Could you check a few things on this model? Use its own coordinates, in mm. A direction names the side the tool comes from. Coordinates: 2 decimals unless noted, no trailing zeros. Loops run counter-clockwise (first coordinate to the right, second up) from the corner with the lowest first, then second, coordinate; pieces in that order, holes last. Notation, with made-up numbers: (54.5, -17.5) - (102.5, -17.5) arc R26 ccw to (102.5, 10.5) - close; hole circle Ø3 at (-20.75, 41). An arc over 180 degrees is marked (long way). Use CSV: the item, a comma, the result in double quotes.
from build123d import *

# Parameters (mm, degrees)
SKETCH1_W           = 80
SKETCH1_H           = 40
BOSS_EXTRUDE1_DEPTH = 100
CUT_EXTRUDE1_DEPTH  = 100
SKETCH4_W           = 20
SKETCH4_H           = 10
CUT_EXTRUDE2_DEPTH  = 100
SKETCH5_W           = 10
SKETCH5_H           = 40
CUT_EXTRUDE3_DEPTH  = 100
SKETCH7_R           = 5
BOSS_EXTRUDE2_DEPTH = 20


with BuildPart() as part:
    # Sketch1 → Boss-Extrude1 (new body)
    with BuildSketch(Plane(origin=(0, 0, 0), x_dir=(1, 0, 0), z_dir=(0, 1, 0))):
        Rectangle(SKETCH1_W, SKETCH1_H)
    extrude(amount=BOSS_EXTRUDE1_DEPTH)

    # Sketch2 → Cut-Extrude1 (cut)
    with BuildSketch(Plane.XY.offset(20)):
        with BuildLine():
            ThreePointArc((20, 30), (34.142135624, 24.142135624), (40, 10))
            Line((40, 10), (40, 100))
            Line((40, 100), (20, 100))
            Line((20, 100), (20, 90))
            ThreePointArc((20, 90), (-10, 60), (20, 30))
        make_face()
        with BuildLine():
            Line((-40, 100), (-40, 70))
            ThreePointArc((-40, 70), (-31.213203436, 91.213203436), (-10, 100))
            Line((-10, 100), (-40, 100))
        make_face()
    extrude(amount=-CUT_EXTRUDE1_DEPTH, mode=Mode.SUBTRACT)

    # Sketch4 → Cut-Extrude2 (cut)
    with BuildSketch(Plane(origin=(40, 0, 0), x_dir=(0, 0, -1), z_dir=(1, 0, 0))):
        with Locations((0, 5)):
            Rectangle(SKETCH4_W, SKETCH4_H)
    extrude(amount=-CUT_EXTRUDE2_DEPTH, mode=Mode.SUBTRACT)

    # Sketch5 → Cut-Extrude3 (cut)
    with BuildSketch(Plane(origin=(20, 0, 0), x_dir=(0, 0, -1), z_dir=(1, 0, 0))):
        with Locations((-15, 80)):
            Rectangle(SKETCH5_W, SKETCH5_H)
    extrude(amount=-CUT_EXTRUDE3_DEPTH, mode=Mode.SUBTRACT)

    # Sketch7 → Boss-Extrude2 (add)
    with BuildSketch(Plane(origin=(0, 0, 0), x_dir=(1, 0, 0), z_dir=(0, 1, 0))):
        with BuildLine():
            Line((10, -20), (-39.600122702, -20))
            ThreePointArc((-39.600122702, -20), (-32.728993539, -22.926933215), (-29.802060324, -29.798062378))
            ThreePointArc((-29.802060324, -29.798062378), (-14.874330774, -50.906091293), (0.33492105, -30))
            ThreePointArc((0.33492105, -30), (3.085632278, -22.987896563), (10, -20))
        make_face()
        with Locations((-14.767737438, -34.998201696)):
            Circle(SKETCH7_R, mode=Mode.SUBTRACT)
    extrude(amount=BOSS_EXTRUDE2_DEPTH)


solid = part.part
(1) Suppose I cut it at C-C (x = 24). Write out the boundary of the cut face in (y, z), plus the area to 3 significant figures.
Computed:
outline,"(0, -20) - (29.6, -20) - (29.6, 20) - (0, 20) - (0, 10) - (10, 10) - (10, -10) - (0, -10) - close"
area,"984 mm²"
(2) Will these pins go through, and if not, where does the flat tip stop? pin 1 (11 mm diameter, centred on x = -13, y = 3.5, fed in from +Z); pin 2 (12 mm diameter, centred on x = -17.5, y = 74.5, fed in from +Z); pin 3 (8 mm diameter, centred on x = -31.5, z = 17, fed in from +Y); pin 4 (11.5 mm diameter, centred on x = -14.77, z = 35, fed in from +Y).
Computed:
pin 1,"stops at z = 50.91"
pin 2,"stops at z = 10"
pin 3,"stops at y = 60"
pin 4,"stops at y = 20"
(3) Thinking about a two-plate mould opening in X: for faces 5 (the face through (40, 5, 15)), 6 (the face through (-16, 80, 10)), 7 (the face through (-18.453, 9.86, 31.619)), which applies, +X half, -X half, draft (parallel to the pull), parting line (faces both ways), or undercut?
Computed:
face 5,"+X half"
face 6,"draft"
face 7,"undercut"
(4) Please list where these lines run through material, in increasing order: line 1 (Z direction, x = 15.5, y = 7); line 2 (Y direction, x = -15, z = 26); line 3 (Z direction, x = 27.5, y = 22.5).
Computed:
line 1,"z = -20 to -10, 10 to 20"
line 2,"y = 0 to 20"
line 3,"z = -20 to 20"
(5) Suppose I cut it at A-A (z = -14). Write out the boundary of the cut face in (x, y).
Computed:
outline,"(-40, 0) - (40, 0) - (40, 10) arc R20 ccw to (20, 30) arc R30 cw to (20, 90) - (20, 100) - (-10, 100) arc R30 ccw to (-40, 70) - close"
(6) Which directions (+Z, -Z, +X, -X, +Y, -Y) give clear straight access to the entire face, cutting with the end or side of a thin tool? Please do faces 1 (the face through (-32.805, 9.86, 22.852)), 2 (the face through (3.011, 9.86, 23.066)), 3 (the face through (1, 5, 10)), 4 (the face through (20, 95, -5)).
Computed:
face 1,"-X, +Y, -Y"
face 2,"+X, +Y, -Y"
face 3,"+X, -X, -Y"
face 4,"+Z, -Z, +X, +Y"
(7) Suppose I cut it at B-B (x = 16). Write out the boundary of the cut face in (y, z), plus the area to 3 significant figures.
Computed:
outline,"(0, -20) - (30.27, -20) - (30.27, 20) - (0, 20) - (0, 10) - (10, 10) - (10, -10) - (0, -10) - close; (89.73, -20) - (100, -20) - (100, 10) - (89.73, 10) - close"
area,"1,320 mm²"
(8) Suppose I cut it at D-D (z = -2). Write out the boundary of the cut face in (x, y).
Computed:
outline,"(-40, 10) - (40, 10) arc R20 ccw to (20, 30) arc R30 cw to (20, 90) - (20, 100) - (-10, 100) arc R30 ccw to (-40, 70) - close"
